from build123d import *

# Parameters (mm, degrees)
SKETCH1_W           = 38.35
SKETCH1_H           = 38.35
BOSS_EXTRUDE1_DEPTH = 1.6
FILLET1_R           = 5
SKETCH2_R           = 1.5
CUT_EXTRUDE1_DEPTH  = 1.6
SKETCH3_W           = 6
SKETCH3_H           = 6
BOSS_EXTRUDE2_DEPTH = 1
SKETCH4_W           = 12
SKETCH4_H           = 8
BOSS_EXTRUDE3_DEPTH = 3


with BuildPart() as part:
    # Sketch1 → Boss-Extrude1 (new body)
    with BuildSketch(Plane(origin=(0, 0, 0), x_dir=(1, 0, 0), z_dir=(0, 1, 0))):
        Rectangle(SKETCH1_W, SKETCH1_H)
    extrude(amount=BOSS_EXTRUDE1_DEPTH)

    # Fillet1
    fillet1_edges = [part.edges().sort_by_distance(p)[0] for p in [
        (19.175, 0.8, 19.175),
        (-19.175, 0.8, 19.175),
        (-19.175, 0.8, -19.175),
        (19.175, 0.8, -19.175),
    ]]
    fillet(fillet1_edges, radius=FILLET1_R)

    # Sketch2 → Cut-Extrude1 (cut)
    with BuildSketch(Plane(origin=(0, 1.6, 0), x_dir=(1, 0, 0), z_dir=(0, 1, 0))):
        with Locations(Location((-14.142135624, 14.142135624, 0), (0, 0, 270))):
            Circle(SKETCH2_R)
        with Locations(Location((14.142135624, 14.142135624, 0), (0, 0, 270))):
            Circle(SKETCH2_R)
        with Locations(Location((-14.142135624, -14.142135624, 0), (0, 0, 270))):
            Circle(SKETCH2_R)
        with Locations(Location((14.142135624, -14.142135624, 0), (0, 0, 270))):
            Circle(SKETCH2_R)
    extrude(amount=-CUT_EXTRUDE1_DEPTH, mode=Mode.SUBTRACT)

    # Sketch3 → Boss-Extrude2 (add)
    with BuildSketch(Plane(origin=(0, 1.6, 0), x_dir=(1, 0, 0), z_dir=(0, 1, 0))):
        Rectangle(SKETCH3_W, SKETCH3_H)
    extrude(amount=BOSS_EXTRUDE2_DEPTH)

    # Sketch4 → Boss-Extrude3 (add)
    with BuildSketch(Plane.XZ):
        with Locations((0, 14.175)):
            Rectangle(SKETCH4_W, SKETCH4_H)
    extrude(amount=BOSS_EXTRUDE3_DEPTH)


solid = part.part
The model under review builds one solid part; all positions refer to its coordinate system, in mm. A direction names the side the tool comes from. Give positions to 0.01 mm unless a question says otherwise; leave off trailing zeros. Loops run counter-clockwise (first coordinate to the right, second up) from the corner with the lowest first, then second, coordinate; pieces in that order, holes last. Notation, with made-up numbers: (22, 19.25) -> (58, 19.25) arc R29 ccw to (58, 53.25) -> close; hole circle Ø11 at (-15, 48). An arc over 180 degrees is marked (long way). Put each result on its own line as item: value. Start each with the question number.
1. We need section D-D on z = -10.5. State the section outline as (x, y) points (3 decimals), then the cut area to 3 significant figures.
2. We need section B-B on y = 1.05. State the section outline as (x, z) points (3 decimals).
3. We need section C-C on z = 12. State the section outline as (x, y) points (3 decimals), then the cut area to 3 significant figures.
4. Wall thickness on probe 1 along Y at (x, z) = (-5, 15); probe 2 along Y at (x, z) = (-4.5, -5); probe 3 along Z at (x, y) = (-5.5, -2.55) (3 decimals): over which ranges is each line inside the solid? List them lowest first.
5. Mouldability with a two-part tool opening along X and no side actions: class faces 1 (the face through (-19.175, 1, 0)), 2 (the face through (-14.72, 0.81, -12.76)), 3 (the face through (17.67, 0.81, 17.75)), 4 (the face through (0, 0, 0)) as released by +X, released by -X, zero draft, split by the parting line, or undercut.
6. We need section A-A on x = -3.5. State the section outline as (y, z) points (3 decimals).
7. For faces 5 (the face through (0, 2, 3)), 6 (the face through (3, 2, 0)), 7 (the face through (-3, 2, 0)), list the 3-axis set-ups (+Z, -Z, +X, -X, +Y, -Y) from which the entire face can be reached by the end or side of a thin tool; tool diameter is ignored.
8. Clearance check with flat-ended pins moving along their axes: P1, Ø4, axis at x = -14.14, z = 14.14, coming from the +Y side; P2, Ø2.5, axis at y = -2, z = 14, coming from the -X side; P3, Ø0.5, axis at x = -0.5, y = 2, coming from the +Z side; P4, Ø1.5, axis at y = -2.5, z = -8.5, coming from the -X side. State where each tip first meets the part, or that it passes through.
Determined:
1. outline: (-19.175, 0) -> (19.175, 0) -> (19.175, 1.6) -> (-19.175, 1.6) -> close
1. area: 61.4 mm^2
2. outline: (-19.175, -14.175) arc R5 ccw to (-14.175, -19.175) -> (14.175, -19.175) arc R5 ccw to (19.175, -14.175) -> (19.175, 14.175) arc R5 ccw to (14.175, 19.175) -> (-14.175, 19.175) arc R5 ccw to (-19.175, 14.175) -> close; hole circle Ø3 at (-14.142, -14.142); hole circle Ø3 at (-14.142, 14.142); hole circle Ø3 at (14.142, -14.142); hole circle Ø3 at (14.142, 14.142)
3. outline: (-19.175, 0) -> (-6, 0) -> (-6, -3) -> (6, -3) -> (6, 0) -> (19.175, 0) -> (19.175, 1.6) -> (-19.175, 1.6) -> close
3. area: 97.4 mm^2
4. probe 1: -3 to 1.6
4. probe 2: 0 to 1.6
4. probe 3: 10.175 to 18.175
5. face 1: released by -X
5. face 2: undercut
5. face 3: released by +X
5. face 4: zero draft
6. outline: (-3, 10.175) -> (0, 10.175) -> (0, -19.175) -> (1.6, -19.175) -> (1.6, 19.175) -> (0, 19.175) -> (0, 18.175) -> (-3, 18.175) -> close
7. face 5: +Z, +X, -X, +Y
7. face 6: +Z, -Z, +X, +Y
7. face 7: +Z, -Z, -X, +Y
8. P1: y = 1.6
8. P2: x = -6
8. P3: z = 3
8. P4: through
